The listing builds one solid part. Answer for the finished solid, in the listing's coordinates (mm). Face numbers are marked on the shaded views. A direction names the side the tool comes from. Give positions to 0.01 mm unless a question says otherwise; leave off trailing zeros. Write each loop counter-clockwise with the first axis right and the second up, starting at its lowest first coordinate (ties: lowest second). Pieces come first, ordered by that corner, then holes. Notation, with made-up numbers: M -24.5,44.25 L 31.5,44.25 A24 ccw 31.5,60.25 Z; hole C 78.5,64 d5. An arc over 180 degrees is marked long. Answer as a JSON object with one key per item and string values.
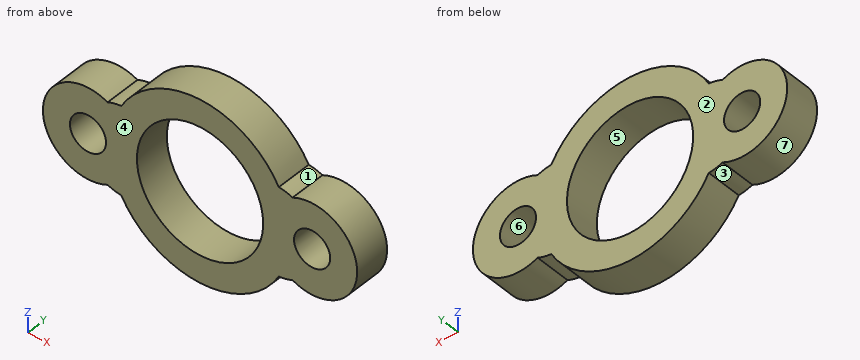
```python
from build123d import *

# Parameters (mm, degrees)
F0_R     = 12.7
F1_DEPTH = 25.4


with BuildPart() as f1:
    # F0 (on Front) → F1 (new body)
    with BuildSketch(Plane.XZ):
        with BuildLine():
            ThreePointArc((-55.4496511867, 30.9448894533), (-61.4544662753, 15.9874505417), (-63.5, 0))
            ThreePointArc((-63.5, 0), (-61.4544662753, -15.9874505417), (-55.4496511867, -30.9448894533))
            ThreePointArc((-55.4496511867, -30.9448894533), (0, -63.5), (55.4496511867, -30.9448894533))
            ThreePointArc((55.4496511867, -30.9448894533), (60.3691549173, -30.174180923), (65.0908594106, -28.5927210679))
            ThreePointArc((65.0908594106, -28.5927210679), (110.6437142577, 0), (65.0908594106, 28.5927210679))
            ThreePointArc((65.0908594106, 28.5927210679), (60.3691549173, 30.174180923), (55.4496511867, 30.9448894533))
            ThreePointArc((55.4496511867, 30.9448894533), (0, 63.5), (-55.4496511867, 30.9448894533))
        make_face()
        with BuildLine():
            ThreePointArc((-44.45, 0), (0, 44.45), (44.45, 0))
            ThreePointArc((44.45, 0), (0, -44.45), (-44.45, 0))
        make_face(mode=Mode.SUBTRACT)
        with BuildLine():
            ThreePointArc((91.5937142577, 0), (78.8937142577, -12.7), (66.1937142577, 0))
            ThreePointArc((66.1937142577, 0), (78.8937142577, 12.7), (91.5937142577, 0))
        make_face(mode=Mode.SUBTRACT)
        with BuildLine():
            ThreePointArc((-55.4496511867, -30.9448894533), (-61.4544662753, -15.9874505417), (-63.5, 0))
            ThreePointArc((-63.5, 0), (-61.4544662753, 15.9874505417), (-55.4496511867, 30.9448894533))
            ThreePointArc((-55.4496511867, 30.9448894533), (-60.3691549173, 30.174180923), (-65.0908594106, 28.5927210679))
            ThreePointArc((-65.0908594106, 28.5927210679), (-110.6437142577, 0), (-65.0908594106, -28.5927210679))
            ThreePointArc((-65.0908594106, -28.5927210679), (-60.3691549173, -30.174180923), (-55.4496511867, -30.9448894533))
        make_face()
        with Locations((-78.8937142577, 0)):
            Circle(F0_R, mode=Mode.SUBTRACT)
    extrude(amount=F1_DEPTH)


solid = f1.part
```
1. A cutting plane is placed at C-C, the plane x = 0. Give the vertices of the cut face in (y, z).
Verdict:
{"outline": "M -25.4,-63.5 L 0,-63.5 L 0,-44.45 L -25.4,-44.45 Z; M -25.4,44.45 L 0,44.45 L 0,63.5 L -25.4,63.5 Z"}
2. A cutting plane is placed at D-D, the plane x = -37. Give the vertices of the cut face in (y, z), plus the area to 3 significant figures.
Verdict:
{"outline": "M -25.4,-51.61 L 0,-51.61 L 0,-24.63 L -25.4,-24.63 Z; M -25.4,24.63 L 0,24.63 L 0,51.61 L -25.4,51.61 Z", "area": "1,370 mm2"}
3. For the marked faces 1, 2 and 3, determine the directions among +Z, -Z, +X, -X, +Y, -Y from which every point of the face is accessible in a straight line to the end or side of a thin tool.
Verdict:
{"face 1": "+Z, +Y, -Y", "face 2": "+Z, -Z, +X, -X, +Y", "face 3": "-Z, +Y, -Y"}
4. The mould has two halves that part along Z. Classify the marked faces 4, 5, 6 and 7: released by +Z, released by -Z, zero draft, split by the parting line, or undercut.
Verdict:
{"face 4": "zero draft", "face 5": "undercut", "face 6": "undercut", "face 7": "split by the parting line"}
5. A cutting plane is placed at B-B, the plane z = 0. Give the vertices of the cut face in (x, y).
Verdict:
{"outline": "M -110.64,-25.4 L -91.59,-25.4 L -91.59,0 L -110.64,0 Z; M -66.19,-25.4 L -44.45,-25.4 L -44.45,0 L -66.19,0 Z; M 44.45,-25.4 L 66.19,-25.4 L 66.19,0 L 44.45,0 Z; M 91.59,-25.4 L 110.64,-25.4 L 110.64,0 L 91.59,0 Z"}
6. Consider line 1 along Z through (x, y) = (0, -18.5); line 2 along X through (y, z) = (-14.25, 7); line 3 along X through (y, z) = (-3, -11). Determine where each line is inside the solid, lowest interval first.
Verdict:
{"line 1": "z = -63.5 to -44.45, 44.45 to 63.5", "line 2": "x = -109.86 to -89.49, -68.3 to -43.9, 43.9 to 68.3, 89.49 to 109.86", "line 3": "x = -108.68 to -85.24, -72.55 to -43.07, 43.07 to 72.55, 85.24 to 108.68"}
7. A cutting plane is placed at A-A, the plane y = -11.25. Give the vertices of the cut face in (x, z), plus the area to 3 significant figures.
Verdict:
{"outline": "M -65.09,-28.59 A29.71 ccw -55.45,-30.94 A63.5 ccw 55.45,-30.94 A29.71 ccw 65.09,-28.59 A31.75 ccw long 65.09,28.59 A29.71 ccw 55.45,30.94 A63.5 ccw -55.45,30.94 A29.71 ccw -65.09,28.59 A31.75 ccw long Z; hole C -78.89,0 d25.4; hole C 0,0 d88.9; hole C 78.89,0 d25.4", "area": "10,800 mm2"}
8. Flat-ended cylindrical pins translate along their axes: pin 1 (12 mm diameter, centred on x = 49, y = -20, fed in from +Z); pin 2 (2 mm diameter, centred on y = -20.5, z = 33.5, fed in from +X); pin 3 (3 mm diameter, centred on y = -5, z = -6.5, fed in from -X). Find the tip coordinate at first contact, or state that the pin passes through.
Verdict:
{"pin 1": "stops at z = 46.73", "pin 2": "stops at x = 54.55", "pin 3": "stops at x = -110.25"}
